from build123d import *

# Parameters (mm, degrees)
F0_R     = 28.575
F1_DEPTH = 3.175
F3_DEPTH = 3.176


# Not quite as in the source:
# - a length typed as a fraction of an inch, garbled in the dataset ("3 / 203.2 mm" for 3/8 in), is restored


with BuildPart() as f1:
    # F0 (on Front) → F1 (new body)
    with BuildSketch(Plane.XZ):
        Circle(F0_R)
    extrude(amount=F1_DEPTH)

    # F2 (on face) → F3 (cut, through all)
    with BuildSketch(Plane.XZ.offset(3.175)):
        with BuildLine():
            Line((-1.75, -17.08304261), (-1.75, -24.075))
            Line((-1.75, -24.075), (0, -24.075))
            Line((0, -24.075), (0, -19.575))
            ThreePointArc((0, -19.575), (-0.9032383957, -18.3488519781), (-1.75, -17.08304261))
        make_face()
        with BuildLine():
            Line((0, -19.575), (0, -24.075))
            Line((0, -24.075), (1.75, -24.075))
            Line((1.75, -24.075), (1.75, -17.2770230976))
            ThreePointArc((1.75, -17.2770230976), (0.9017072988, -18.4463502097), (0, -19.575))
        make_face()
        with BuildLine():
            ThreePointArc((-6.9936556862, 0), (-5.528073584, -8.8964320017), (-1.75, -17.08304261))
            ThreePointArc((-1.75, -17.08304261), (-0.9032383957, -18.3488519781), (0, -19.575))
            Line((0, -19.575), (0, 0))
            Line((0, 0), (-6.9936556862, 0))
        make_face()
        with BuildLine():
            Line((0, 0), (0, -19.575))
            ThreePointArc((0, -19.575), (0.9017072988, -18.4463502097), (1.75, -17.2770230976))
            ThreePointArc((1.75, -17.2770230976), (5.789623043, -9.0487471984), (7.2536082684, 0))
            Line((7.2536082684, 0), (0, 0))
        make_face()
        with BuildLine():
            ThreePointArc((-6, 9.1323722154), (-6.8103344804, 4.6002974695), (-6.9936556862, 0))
            Line((-6.9936556862, 0), (0, 0))
            Line((0, 0), (7.2536082684, 0))
            ThreePointArc((7.2536082684, 0), (6.9672213091, 4.6129154541), (6, 9.1323722154))
            Line((6, 9.1323722154), (6, 18.5192639611))
            Line((6, 18.5192639611), (9.3, 18.5192639611))
            Line((9.3, 18.5192639611), (9.3, 27.0192639611))
            ThreePointArc((9.3, 27.0192639611), (0, 28.575), (-9.3, 27.0192639611))
            Line((-9.3, 27.0192639611), (-9.3, 18.5192639611))
            Line((-9.3, 18.5192639611), (-6, 18.5192639611))
            Line((-6, 18.5192639611), (-6, 9.1323722154))
        make_face()
        with BuildLine():
            Line((12.5375, 0), (16.0375, 0))
            Line((16.0375, 0), (16.0375, 23.650142045))
            ThreePointArc((16.0375, 23.650142045), (14.3234197578, 24.7259028438), (12.5375, 25.6776501797))
            Line((12.5375, 25.6776501797), (12.5375, 0))
        make_face()
        with BuildLine():
            Line((-16.0375, 0), (-12.5375, 0))
            Line((-12.5375, 0), (-12.5375, 25.6776501797))
            ThreePointArc((-12.5375, 25.6776501797), (-14.3234197578, 24.7259028438), (-16.0375, 23.650142045))
            Line((-16.0375, 23.650142045), (-16.0375, 0))
        make_face()
    extrude(amount=-F3_DEPTH, mode=Mode.SUBTRACT)


solid = f1.part
Can you work these out from the model? Positions are in its coordinate system, mm. A direction names the side the tool comes from. Round coordinates to 2 decimals unless told otherwise and drop trailing zeros. Order: outer loops, then holes, each group sorted by start corner. A loop starts at its lowest first (then second) coordinate and runs counter-clockwise, first axis right, second up. Notation, with made-up numbers: (63, -21.5) -> (96, -21.5) arc R33 cw to (96, 11.5) -> close; hole circle Ø11 at (70, 57). An arc over 180 degrees is marked (long way). Write each question's results on one line, items separated by ' | '. Start each with the question number.
Item 1: Will these pins go through, and if not, where does the flat tip stop? pin 1 (1 mm diameter, centred on x = 14, y = -1, fed in from +Z); pin 2 (1 mm diameter, centred on y = -1.5, z = 13.5, fed in from +X); pin 3 (1.6 mm diameter, centred on y = -2, z = 25, fed in from +X); pin 4 (1.5 mm diameter, centred on x = 5, z = 6.5, fed in from +Y).
Item 2: If we section it at D-D, the plane x = 0: Write out the boundary of the cut face in (y, z) (3 decimals), then the cut area to 3 significant figures.
Item 3: If we section it at A-A, the plane z = -22: Write out the boundary of the cut face in (x, y) (3 decimals).
Item 4: If we section it at B-B, the plane z = 6.5: Write out the boundary of the cut face in (x, y) (1 decimal).
Item 5: Please list where these lines run through material, in increasing order: L1, parallel to X at y = -0.4, z = 7.5; L2, parallel to X at y = -0.6, z = 20; L3, parallel to X at y = -0.9, z = -20.
Item 6: Which directions (+Z, -Z, +X, -X, +Y, -Y) give clear straight access to the entire face, cutting with the end or side of a thin tool? Please do faces 1 (the cylindrical face through (10.96, -1.57, 26.39)), 2 (the flat face through (0, -2, -24.075)).
Results:
1) pin 1: stops at z = 0 | pin 2: stops at x = 25.45 | pin 3: stops at x = 12.54 | pin 4: passes through
2) outline: (-3.175, -28.575) -> (0, -28.575) -> (0, -24.075) -> (-3.175, -24.075) -> close | area: 14.3 mm2
3) outline: (-18.235, -3.175) -> (-1.75, -3.175) -> (-1.75, 0) -> (-18.235, 0) -> close; (1.75, -3.175) -> (18.235, -3.175) -> (18.235, 0) -> (1.75, 0) -> close
4) outline: (-27.8, -3.2) -> (-16, -3.2) -> (-16, 0) -> (-27.8, 0) -> close; (-12.5, -3.2) -> (-6.5, -3.2) -> (-6.5, 0) -> (-12.5, 0) -> close; (6.6, -3.2) -> (12.5, -3.2) -> (12.5, 0) -> (6.6, 0) -> close; (16, -3.2) -> (27.8, -3.2) -> (27.8, 0) -> (16, 0) -> close
5) L1: x = -27.57 to -16.04, -12.54 to -6.37, 6.43 to 12.54, 16.04 to 27.57 | L2: x = -20.41 to -16.04, -12.54 to -9.3, 9.3 to 12.54, 16.04 to 20.41 | L3: x = -20.41 to -1.75, 1.75 to 20.41
6) face 1: +Z, +X, +Y, -Y | face 2: +Z, +Y, -Y
